Print and shaded views of the part. All mm, measured from the part's lowest x, y and z. A direction names the side the tool comes from. Give positions to 0.01 mm unless a question says otherwise; leave off trailing zeros. Order: outer loops, then holes, each group sorted by start corner. A loop starts at its lowest first (then second) coordinate and runs counter-clockwise, first axis right, second up. Notation, with made-up numbers: (48.25, 48.25) -> (96.25, 48.25) arc R27 cw to (96.25, 79.25) -> close; hole circle Ø11 at (-30, 35). An arc over 180 degrees is marked (long way). One line per question, with ' | ' between items. Start each with the question number.
(1) Cut at A-A (z = 32.5). Give the cut face in (x, y), then the cut area to 3 significant figures.
(2) Which spindle directions (+Z, -Z, +X, -X, +Y, -Y) get a long thin tool onto all of the face, cutting with end or side? Do the marked faces 4, 5 and 6. Say none if no direction does.
(3) Pull direction Y, two halves, no side cores. Call the marked faces 1, 2 and 3: +Y half, -Y half, draft (parallel to the pull), parting line (faces both ways), or undercut.
(4) Drill centre lines: L1, parallel to Z at x = 26.5, y = 24.5; L2, parallel to Z at x = 15.5, y = 34; L3, parallel to Y at x = 22.5, z = 36. Where is each one in solid material? Low to high. Write a range as from..to.
(5) Pin check, flat tips, straight feed: pin 1 Ø8 at (y, z) = (33, 6.5) entering from +X; pin 2 Ø8 at (x, z) = (35, 29) entering from +Y; pin 3 Ø7.5 at (x, y) = (23.5, 23.5) entering from +Z. Stop position of each tip, or through.
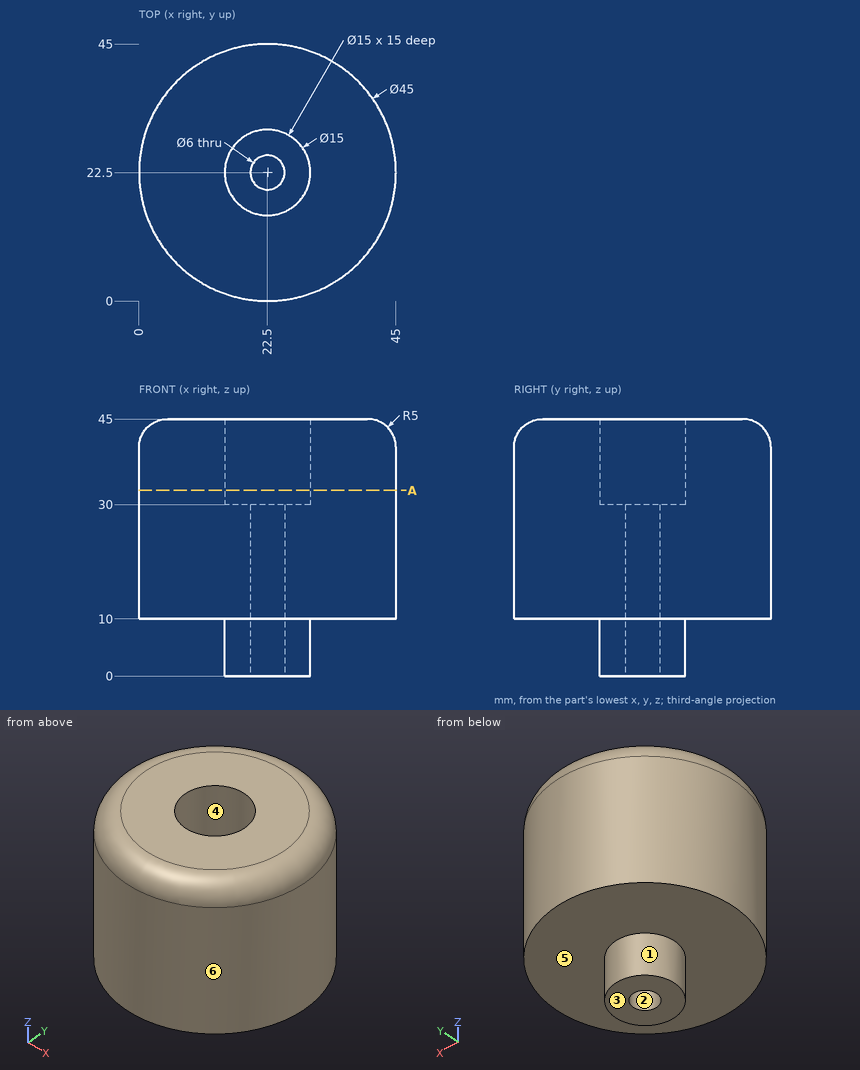
Result set:
1) outline: circle Ø45 at (22.5, 22.5); hole circle Ø15 at (22.5, 22.5) | area: 1,410 mm2
2) face 4: +Z | face 5: -Z | face 6: +Z, -Z
3) face 1: parting line | face 2: undercut | face 3: draft
4) L1: z = 0..30 | L2: z = 10..45 | L3: y = 0..15, 30..45
5) pin 1: stops at x = 43.31 | pin 2: stops at y = 43.33 | pin 3: stops at z = 30
